Source: CAD feature listing. Evaluate the final solid. Frame: model axes, mm. Round coordinates to 2 decimals unless told otherwise and drop trailing zeros. Loops run counter-clockwise (first coordinate to the right, second up) from the corner with the lowest first, then second, coordinate; pieces in that order, holes last.
(1) Material intervals for probe 1 along X at (y, z) = (-50.6, 0.7); probe 2 along Y at (x, z) = (44.5, 1) (3 decimals); probe 3 along X at (y, z) = (-51, 1.05), sorted ascending.
(2) Section B-B, the plane y = -48.15. Return the cut outline in (x, z), plus the area to 3 significant figures.
(3) Section A-A, the plane z = 1.2. Return the cut outline in (x, y) (3 decimals).
(4) First-contact query: pin 1 Ø1 at (y, z) = (-53, 1.5) entering from -X. Flat tip, straight axial feed; report the tip coordinate or a pass-through.
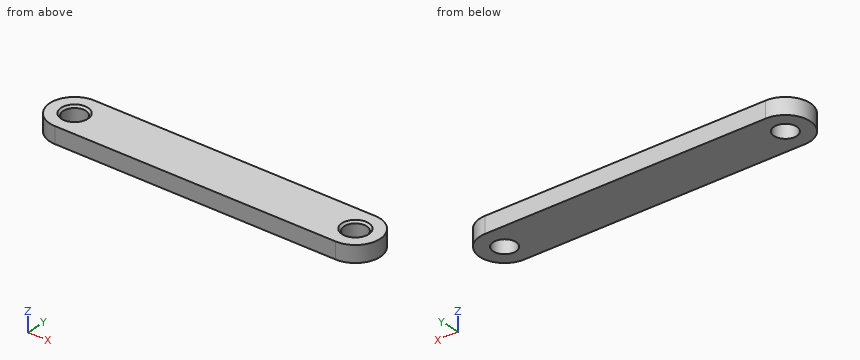
```python
from build123d import *

# Parameters (mm, degrees)
SKETCH1_R           = 1.375
BOSS_EXTRUDE1_DEPTH = 2
CHAMFER1_SIZE       = 0.25


with BuildPart() as part:
    # Sketch1 → Boss-Extrude1 (new body)
    with BuildSketch(Plane.XY):
        with BuildLine():
            Line((44.5, -47.65), (10.5, -47.65))
            ThreePointArc((10.5, -47.65), (7.5, -50.65), (10.5, -53.65))
            Line((10.5, -53.65), (44.5, -53.65))
            ThreePointArc((44.5, -53.65), (47.5, -50.65), (44.5, -47.65))
        make_face()
        with Locations((10.5, -50.65)):
            Circle(SKETCH1_R, mode=Mode.SUBTRACT)
        with Locations((44.5, -50.65)):
            Circle(SKETCH1_R, mode=Mode.SUBTRACT)
    extrude(amount=BOSS_EXTRUDE1_DEPTH)

    # Chamfer1
    chamfer1_edges = [part.edges().sort_by_distance(p)[0] for p in [
        (9.125, -50.65, 2),
        (43.125, -50.65, 2),
    ]]
    chamfer(chamfer1_edges, length=CHAMFER1_SIZE)


solid = part.part
```
Output values:
1. probe 1: x = 7.5 to 9.13, 11.87 to 43.13, 45.87 to 47.5
1. probe 2: y = -53.65 to -52.025, -49.275 to -47.65
1. probe 3: x = 7.52 to 9.17, 11.83 to 43.17, 45.83 to 47.48
2. outline: (8.84, 0) - (46.16, 0) - (46.16, 2) - (8.84, 2) - close
2. area: 74.6 mm2
3. outline: (10.5, -53.65) - (44.5, -53.65) arc R3 ccw to (44.5, -47.65) - (10.5, -47.65) arc R3 ccw to start; hole circle Ø2.75 at (10.5, -50.65); hole circle Ø2.75 at (44.5, -50.65)
4. pin 1: stops at x = 8.14
